from build123d import *

# Parameters (mm, degrees)
F1_DEPTH    = 20
F2_T1_DEPTH = 125.4092553389
F3_D        = 10
F3_DEPTH    = 10
F3_TIP      = 3.0043030951
F4_R        = 18
F5_DEPTH    = 30
F7_D        = 14
F7_DEPTH    = 31
F7_TIP      = 4.2060243332
F8_T1_DEPTH = 79.2927061282


# Not quite as in the source:
# - a fillet or chamfer that OpenCascade refuses, or shapes differently, is made with other operations: its cross-section is extruded or revolved along the edge and cut away or added


with BuildPart() as f1:
    # F0 (on Front) → F1 (new body)
    with BuildSketch(Plane.XZ):
        with BuildLine():
            ThreePointArc((10.7142859294, -22.5876974706), (21.1288564318, -13.363061995), (25, 0))
            ThreePointArc((25, 0), (21.1288563814, 13.3630620747), (10.7142857589, 22.5876975515))
            ThreePointArc((10.7142857589, 22.5876975515), (1.61e-08, 25), (-10.7142857298, 22.5876975653))
            ThreePointArc((-10.7142857298, 22.5876975653), (-21.1288563728, 13.3630620884), (-25, 0))
            ThreePointArc((-25, 0), (-21.1288561313, -13.3630624702), (-10.7142849134, -22.5876979525))
            ThreePointArc((-10.7142849134, -22.5876979525), (5.623e-07, -25), (10.7142859294, -22.5876974706))
        make_face()
        with BuildLine():
            ThreePointArc((-39.2857140137, -9.0350791581), (-45, -4.32e-08), (-39.2857140918, 9.035079121))
            Line((-39.2857140918, 9.035079121), (-58.3333333333, 0))
            Line((-58.3333333333, 0), (-39.2857140137, -9.0350791581))
        make_face()
        with BuildLine():
            ThreePointArc((-25, 0), (-21.1288563728, 13.3630620884), (-10.7142857298, 22.5876975653))
            Line((-10.7142857298, 22.5876975653), (-39.2857140918, 9.035079121))
            ThreePointArc((-39.2857140918, 9.035079121), (-29.6547750711, 8.4515424899), (-25, 0))
        make_face()
        with BuildLine():
            Line((-39.2857140137, -9.0350791581), (-10.7142849134, -22.5876979525))
            ThreePointArc((-10.7142849134, -22.5876979525), (-21.1288561313, -13.3630624702), (-25, 0))
            ThreePointArc((-25, 0), (-29.6547750345, -8.4515424668), (-39.2857140137, -9.0350791581))
        make_face()
        with BuildLine():
            ThreePointArc((-39.2857140137, -9.0350791581), (-29.6547750345, -8.4515424668), (-25, 0))
            ThreePointArc((-25, 0), (-29.6547750711, 8.4515424899), (-39.2857140918, 9.035079121))
            ThreePointArc((-39.2857140918, 9.035079121), (-45, -4.32e-08), (-39.2857140137, -9.0350791581))
        make_face()
        with BuildLine():
            Line((0, -27.6699295265), (10.7142859294, -22.5876974706))
            ThreePointArc((10.7142859294, -22.5876974706), (5.623e-07, -25), (-10.7142849134, -22.5876979525))
            Line((-10.7142849134, -22.5876979525), (0, -27.6699295265))
        make_face()
        with BuildLine():
            ThreePointArc((-10.7142857298, 22.5876975653), (1.61e-08, 25), (10.7142857589, 22.5876975515))
            Line((10.7142857589, 22.5876975515), (0, 27.6699295265))
            Line((0, 27.6699295265), (-10.7142857298, 22.5876975653))
        make_face()
        with BuildLine():
            Line((58.3333333333, 0), (39.2857143013, 9.0350790217))
            ThreePointArc((39.2857143013, 9.0350790217), (43.4515425519, 5.345224831), (45, 0))
            ThreePointArc((45, 0), (43.4515424899, -5.3452249289), (39.2857140918, -9.035079121))
            Line((39.2857140918, -9.035079121), (58.3333333333, 0))
        make_face()
        with BuildLine():
            ThreePointArc((10.7142857589, 22.5876975515), (21.1288563814, 13.3630620747), (25, 0))
            ThreePointArc((25, 0), (29.654775169, 8.4515425519), (39.2857143013, 9.0350790217))
            Line((39.2857143013, 9.0350790217), (10.7142857589, 22.5876975515))
        make_face()
        with BuildLine():
            ThreePointArc((39.2857140918, -9.035079121), (29.6547750711, -8.4515424899), (25, 0))
            ThreePointArc((25, 0), (21.1288564318, -13.363061995), (10.7142859294, -22.5876974706))
            Line((10.7142859294, -22.5876974706), (39.2857140918, -9.035079121))
        make_face()
        with BuildLine():
            ThreePointArc((39.2857143013, 9.0350790217), (29.654775169, 8.4515425519), (25, 0))
            ThreePointArc((25, 0), (29.6547750711, -8.4515424899), (39.2857140918, -9.035079121))
            ThreePointArc((39.2857140918, -9.035079121), (43.4515424899, -5.3452249289), (45, 0))
            ThreePointArc((45, 0), (43.4515425519, 5.345224831), (39.2857143013, 9.0350790217))
        make_face()
    extrude(amount=-F1_DEPTH)

    # F2: fillet of radius 10 on 2 edges, made by hand

    # F2_s2 → F2_t1 (cut)
    with BuildSketch(Plane.XZ.offset(-72.7046276695)):
        with BuildLine():
            ThreePointArc((-39.2857142857, -9.0350790291), (-45, 0), (-39.2857142857, 9.0350790291))
            Line((-39.2857142857, 9.0350790291), (-58.3333333333, 0))
            Line((-58.3333333333, 0), (-39.2857142857, -9.0350790291))
        make_face()
        with BuildLine():
            ThreePointArc((39.2857142857, -9.0350790291), (45, 0), (39.2857142857, 9.0350790291))
            Line((39.2857142857, 9.0350790291), (58.3333333333, 0))
            Line((58.3333333333, 0), (39.2857142857, -9.0350790291))
        make_face()
    extrude(amount=F2_T1_DEPTH, mode=Mode.SUBTRACT)

    # F3
    with Locations(Plane.XZ):
        with Locations((-35, 0), (35, 0)):
            Hole(F3_D / 2, depth=F3_DEPTH)
            with Locations((0, 0, -(F3_DEPTH + F3_TIP / 2))):  # 118° drill point
                Cone(0, F3_D / 2, F3_TIP, mode=Mode.SUBTRACT)

    # F4 (on face) → F5 (join)
    with BuildSketch(Plane.XZ):
        Circle(F4_R)
    extrude(amount=F5_DEPTH)

    # F7
    with Locations(Plane.XZ.offset(30)):
        with Locations((0, 0)):
            Hole(F7_D / 2, depth=F7_DEPTH)
            with Locations((0, 0, -(F7_DEPTH + F7_TIP / 2))):  # 118° drill point
                Cone(0, F7_D / 2, F7_TIP, mode=Mode.SUBTRACT)

    # F8: fillet of radius 25 on 2 edges, made by hand

    # F8_s2 → F8_t1 (cut)
    with BuildSketch(Plane.XZ.offset(-49.6463530641)):
        with BuildLine():
            ThreePointArc((-10.7142857143, 22.5876975726), (0, 25), (10.7142857143, 22.5876975726))
            Line((10.7142857143, 22.5876975726), (0, 27.6699295265))
            Line((0, 27.6699295265), (-10.7142857143, 22.5876975726))
        make_face()
        with BuildLine():
            ThreePointArc((-10.7142857143, -22.5876975726), (0, -25), (10.7142857143, -22.5876975726))
            Line((10.7142857143, -22.5876975726), (0, -27.6699295265))
            Line((0, -27.6699295265), (-10.7142857143, -22.5876975726))
        make_face()
    extrude(amount=F8_T1_DEPTH, mode=Mode.SUBTRACT)


solid = f1.part
The listing builds one solid part. Answer for the finished solid, in the listing's coordinates (mm). A direction names the side the tool comes from. Round coordinates to 2 decimals unless told otherwise and drop trailing zeros. Loops run counter-clockwise (first coordinate to the right, second up) from the corner with the lowest first, then second, coordinate; pieces in that order, holes last. Notation, with made-up numbers: M -3,-30 L 37,-30 A10 cw 37,-18 Z; hole C 33.5,-28.75 d11. An arc over 180 degrees is marked long. Write each question's results on one line, items separated by ' | '. Start each with the question number.
1) Find section D-D on z = -11.5. Write down the section's boundary in (x, y).
2) Determine the mould class of faces 1 (the cylindrical face through (-2.343, -14.79, 17.847)), 2 (the flat face through (-1, 20, 0)), 3 (the conical face through (34.31, 12.48, -0.53)) for opening direction Z: pulls with the +Z half, pulls with the -Z half, needs draft (parallel to the pull), parting line crosses it, or undercut.
3) Each of these flat-tipped pins is pushed along its axis until it touches: pin 1 (12 mm diameter, centred on x = -3.5, y = -15, fed in from -Z); pin 2 (11 mm diameter, centred on x = 0, z = 0, fed in from -Y); pin 3 (12 mm diameter, centred on x = -0.5, y = -8.5, fed in from +Z). Where does it stop, or does it pass through?
4) Find section A-A on y = -20. Write down the section's boundary in (x, z), plus the area to 3 significant figures.
5) Which of the six approach directions +Z, -Z, +X, -X, +Y, -Y give full straight-line access (tool end or side, diameter ignored) to faces 4 (the cylindrical face through (0, 10, -25)), 5 (the cylindrical face through (-30, 5, 0))?
6) Find section C-C on x = 29. Write down the section's boundary in (y, z), plus the area to 3 significant figures.
7) Find section B-B on z = 16. Write down the section's boundary in (x, y), plus the area to 3 significant figures.
8) Straight lines are drawn through the part: probe 1 along Z at (x, y) = (0, -16); probe 2 along X at (y, z) = (3, 2); probe 3 along Y at (x, z) = (-10, 22.5). For each, find the intervals that lie inside material, in ascending order.
Final values:
1) outline: M -34.09,0 L -13.85,0 L -13.85,-30 L 13.85,-30 L 13.85,0 L 34.09,0 L 34.09,20 L -34.09,20 Z
2) face 1: parting line crosses it | face 2: needs draft | face 3: undercut
3) pin 1: z = -18 | pin 2: y = 1.9 | pin 3: z = 18
4) outline: C 0,0 d36; hole C 0,0 d14 | area: 864 mm²
5) face 4: -Z, +Y, -Y | face 5: -Y
6) outline: M 0,-13.91 L 20,-13.91 L 20,13.91 L 0,13.91 Z | area: 557 mm²
7) outline: M -24.6,0 L -8.25,0 L -8.25,-30 L 8.25,-30 L 8.25,0 L 24.6,0 L 24.6,20 L -24.6,20 Z | area: 1,480 mm²
8) probe 1: -18 to -7, 7 to 18 | probe 2: -44.8 to -39.58, -30.42 to -3.08, 3.08 to 30.42, 39.58 to 44.8 | probe 3: 0 to 20
